from build123d import *

# Parameters (mm, degrees)
F3_D            = 8.5
F3_COPIES_COUNT = 20


# Not quite as in the source:
# - a pattern or mirror of a feature is missing from the dataset's text; its kind, count and spacing are read off the source's solid


with BuildPart() as f1:
    # F0 (on Front) → F1 (revolve)
    with BuildSketch(Plane.XZ):
        with BuildLine():
            Line((40, 310), (40, 112.5))
            ThreePointArc((40, 112.5), (54.6446609407, 77.1446609407), (90, 62.5))
            Line((90, 62.5), (100, 62.5))
            Line((100, 62.5), (100, 72.5))
            Line((100, 72.5), (90, 72.5))
            ThreePointArc((90, 72.5), (61.7157287525, 84.2157287525), (50, 112.5))
            Line((50, 112.5), (50, 320))
            Line((50, 320), (10, 320))
            Line((10, 320), (10, 360))
            Line((10, 360), (0, 360))
            Line((0, 360), (0, 310))
            Line((0, 310), (40, 310))
        make_face()
    revolve(axis=Axis((50, 0, 0), (1, 0, 0)))

    # F3 (through all)
    with Locations(Plane.YZ.offset(10)):
        with Locations((0, 340)):
            f3 = Hole(F3_D / 2)

    # F3_copies: F3 ×20 about axis
    f3_copies_axis = Axis((0, 0, 0), (1, 0, 0))
    for i in range(1, F3_COPIES_COUNT):
        add(f3.rotate(f3_copies_axis, i * 360 / F3_COPIES_COUNT), mode=Mode.SUBTRACT)


solid = f1.part
Verification items for the finished model (mm, model axes). A direction names the side the tool comes from. Round coordinates to 2 decimals unless told otherwise and drop trailing zeros. Order: outer loops, then holes, each group sorted by start corner. A loop starts at its lowest first (then second) coordinate and runs counter-clockwise, first axis right, second up. Notation, with made-up numbers: (44.5, 58.25) -> (51.5, 58.25) arc R19 ccw to (51.5, 88.25) -> close; hole circle Ø3 at (22.5, 65). An arc over 180 degrees is marked (long way). Put each result on its own line as item: value.
1) Depth check by flat-ended pin: pin 1 (10 mm diameter, centred on y = 105.07, z = -323.36, fed in from +X); pin 2 (10 mm diameter, centred on y = 0, z = -340, fed in from -X); pin 3 (2 mm diameter, centred on y = 192, z = -165.5, fed in from +X); pin 4 (4 mm diameter, centred on x = 31.5, z = -154.5, fed in from +Y) (3 decimals). Enter the tip coordinate at first touch or a pass-through.
Final values:
pin 1: stops at x = 10
pin 2: stops at x = 0
pin 3: stops at x = 50
pin 4: stops at y = 281.325
2) Section check C-C (y = -289). Record the cut outline in (x, z), then the cut area to 3 significant figures.
Final values:
outline: (0, -214.66) -> (10, -214.66) -> (10, -137.4) -> (50, -137.4) -> (50, 137.4) -> (10, 137.4) -> (10, 214.66) -> (0, 214.66) -> (0, 112.16) -> (40, 112.16) -> (40, -112.16) -> (0, -112.16) -> close
area: 6,310 mm^2
3) Section check B-B (x = 69.5). Record the cut outline in (y, z).
Final values:
outline: circle Ø156.31 at (0, 0); hole circle Ø133.79 at (0, 0)
4) Mould release check, pull along Y, two halves, no side actions. Record for faces 4 (the cylindrical face through (29.72, 312.39, -69.37)), 5 (the flat face through (100, -54, -32)), 6 (the flat face through (40, -4, 133)): +Y half, -Y half, draft (parallel to the pull), parting line (faces both ways), or undercut.
Final values:
face 4: parting line
face 5: draft
face 6: undercut
5) Material ranges on line 1 (Z direction, x = 5.25, y = 0); line 2 (Z direction, x = 38, y = 5); line 3 (X direction, y = -96.5, z = -176.5), recorded low to high.
Final values:
line 1: z = -360 to -344.25, -335.75 to -310, 310 to 335.75, 344.25 to 360
line 2: z = -319.96 to -309.96, 309.96 to 319.96
line 3: x = 40 to 50
6) Set-up check for faces 1 (the cylindrical face through (4.93, 319.38, 166.12)), 2 (the flat face through (10, -322, 2)), 3 (the cylindrical face through (20.28, 302.63, -67.2)): record each of +Z, -Z, +X, -X, +Y, -Y from which the full face is reachable in a straight line by a thin tool's end or side.
Final values:
face 1: +X, -X
face 2: +X
face 3: -X
7) Section check A-A (y = -125). Record the cut outline in (x, z).
Final values:
outline: (0, -337.6) -> (10, -337.6) -> (10, -294.58) -> (50, -294.58) -> (50, 294.58) -> (10, 294.58) -> (10, 337.6) -> (0, 337.6) -> (0, 283.68) -> (40, 283.68) -> (40, -283.68) -> (0, -283.68) -> close
